```python
from build123d import *

# Parameters (mm, degrees)
SKETCH1_R           = 7
BOSS_EXTRUDE1_DEPTH = 10
RIB1_REACH          = 79.589
SKETCH2_WALL_W      = 192.003076928
SKETCH2_WALL_H      = 6
SKETCH3_R           = 2.5
CUT_EXTRUDE1_DEPTH  = 65.031242374


with BuildPart() as part:
    # Sketch1 → Boss-Extrude1 (new, symmetric)
    with BuildSketch(Plane.YZ):
        with BuildLine():
            Line((26.324893162, 3), (40.167603026, 3))
            ThreePointArc((40.167603026, 3), (41.844654009, 3.512531407), (42.948677458, 4.875))
            ThreePointArc((42.948677458, 4.875), (68, 0), (42.948677458, -4.875))
            ThreePointArc((42.948677458, -4.875), (41.844654009, -3.512531407), (40.167603026, -3))
            Line((40.167603026, -3), (26.324893162, -3))
            ThreePointArc((26.324893162, -3), (24.454064469, -3.65479212), (23.399905033, -5.333333333))
            ThreePointArc((23.399905033, -5.333333333), (20.675987443, -12.186202988), (16, -17.88854382))
            Line((16, -17.88854382), (16, -36))
            Line((16, -36), (2.5, -36))
            Line((2.5, -36), (2.5, -15.803480629))
            ThreePointArc((2.5, -15.803480629), (0, 16), (-2.5, -15.803480629))
            Line((-2.5, -15.803480629), (-2.5, -36))
            Line((-2.5, -36), (-16, -36))
            Line((-16, -36), (-16, -17.88854382))
            ThreePointArc((-16, -17.88854382), (-12.186202988, 20.675987443), (23.399905033, 5.333333333))
            ThreePointArc((23.399905033, 5.333333333), (24.454064469, 3.65479212), (26.324893162, 3))
        make_face()
        with Locations(Location((55, 0, 0), (0, 0, 270))):
            Circle(SKETCH1_R, mode=Mode.SUBTRACT)
    extrude(amount=BOSS_EXTRUDE1_DEPTH, both=True)

    # Sketch2 wall → Rib1 (add, up to next)
    with BuildSketch(Plane(origin=(0, 37.587120501, 13), x_dir=(0, -1, 0), z_dir=(0, 0, -1)), mode=Mode.PRIVATE) as rib1_sk1:
        Rectangle(SKETCH2_WALL_W, SKETCH2_WALL_H)
    rib1_tool1 = extrude(rib1_sk1.sketch, amount=RIB1_REACH, mode=Mode.PRIVATE) - part.part
    add(rib1_tool1.solids().sort_by_distance((0, 37.587120501, 13))[0])

    # Sketch3 → Cut-Extrude1 (cut, through all)
    with BuildSketch(Plane(origin=(0, 16, 0), x_dir=(-1, 0, 0), z_dir=(0, 1, 0))):
        with Locations(Location((0, -27, 0), (0, 0, 90))):
            Circle(SKETCH3_R)
    extrude(amount=-CUT_EXTRUDE1_DEPTH, mode=Mode.SUBTRACT)


solid = part.part
```
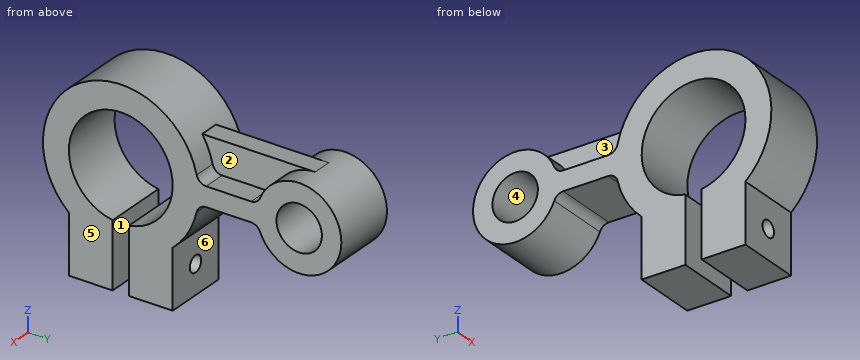
Geometry: final body of the model. Coordinates: model frame, mm. Face numbers are marked on the shaded views. A direction names the side the tool comes from. Round coordinates to 2 decimals unless told otherwise and drop trailing zeros. Order: outer loops, then holes, each group sorted by start corner. A loop starts at its lowest first (then second) coordinate and runs counter-clockwise, first axis right, second up. Notation, with made-up numbers: M -20,6.25 L -10,6.25 A18 ccw -10,13.25 Z; hole C 14,63 d11. An arc over 180 degrees is marked long. Use one line per item in the form item = value. Start each with the question number.
Q1. Cut plane B-B (z = 0). Return loops of the section in (x, y).
Q2. Mould query, pull axis Y, two halves, no side actions, for the marked faces 4, 5 and 6. Classes: +Y half, -Y half, draft (parallel to the pull), parting line (faces both ways), or undercut.
Q3. Pin query (flat end, axial travel): pin 1 Ø3.5 at (x, y) = (6, 32.5) entering from +Z; pin 2 Ø10 at (x, z) = (1.5, -24.5) entering from -Y; pin 3 Ø3 at (x, z) = (0, -27) entering from -Y; pin 4 Ø2 at (x, y) = (0.5, 17.5) entering from -Z. Return the tip coordinate at first contact, or that it passes through.
Q4. Cut plane C-C (z = -23). Return loops of the section in (x, y), and give its area (3 significant figures).
Q5. Access query for the marked faces 1, 2 and 3. Directions: +Z, -Z, +X, -X, +Y, -Y. A direction counts if a zero-diameter tool reaches every point of the face in a straight line with its end or side. Return the directions, or none.
Q6. Cut plane A-A (x = 0). Return loops of the section in (y, z) (3 decimals).
Q7. Cut plane D-D (x = 6). Return loops of the section in (y, z) (3 decimals).
Q8. Material intervals for line 1 (Y direction, x = 4.75, z = 10); line 2 (X direction, y = -11, z = -27); line 3 (Y direction, x = 6.5, z = -29), sorted ascending. Write a range as [from, to].
Geometry results:
q1.outline = M -10,-24 L 10,-24 L 10,-16 L -10,-16 Z; M -10,16 L 10,16 L 10,48 L -10,48 Z; M -10,62 L 10,62 L 10,68 L -10,68 Z
q2.face_4 = undercut
q2.face_5 = draft
q2.face_6 = +Y half
q3.pin_1 = 3
q3.pin_2 = -16
q3.pin_3 = through
q3.pin_4 = -17.43
q4.outline = M -10,-16 L 10,-16 L 10,-2.5 L -10,-2.5 Z; M -10,2.5 L 10,2.5 L 10,16 L -10,16 Z
q4.area = 540 mm^2
q5.face_1 = -Z, +X, -X
q5.face_2 = +Z, +X
q5.face_3 = +Z, -X
q6.outline = M -16,-36 L -2.5,-36 L -2.5,-29.5 L -16,-29.5 Z; M -16,-24.5 L -2.5,-24.5 L -2.5,-15.803 A16 cw long 2.5,-15.803 L 2.5,-24.5 L 16,-24.5 L 16,-17.889 A24 ccw 23.4,-5.333 A3 cw 26.325,-3 L 40.168,-3 A3 cw 42.949,-4.875 A13 ccw long 55,13 L 20.174,13 A24 ccw long -16,-17.889 Z; M 2.5,-36 L 16,-36 L 16,-29.5 L 2.5,-29.5 Z; hole C 55,0 d14
q7.outline = M -16,-36 L -2.5,-36 L -2.5,-15.803 A16 cw long 2.5,-15.803 L 2.5,-36 L 16,-36 L 16,-17.889 A24 ccw 23.4,-5.333 A3 cw 26.325,-3 L 40.168,-3 A3 cw 42.949,-4.875 A13 ccw long 42.949,4.875 A3 cw 40.168,3 L 26.325,3 A3 cw 23.4,5.333 A24 ccw long -16,-17.889 Z; hole C 55,0 d14
q8.line_1 = [-21.82, -12.49], [12.49, 21.82], [46.69, 63.31]
q8.line_2 = [-10, -2.5], [2.5, 10]
q8.line_3 = [-16, -2.5], [2.5, 16]
